from build123d import *

# Parameters (mm, degrees)
F0_R     = 3
F1_DEPTH = 6
F2_R     = 8.6602540378
F3_DEPTH = 6
F4_R     = 5.99999
F5_R     = 0.75
F6_DEPTH = 3
F7_R     = 3
F8_DEPTH = 101
F10_R    = 2.5
F11_R    = 3


# Not quite as in the source:
# - a fillet or chamfer is up to 0.001 mm smaller than in the source, because OpenCascade refuses the exact size


with BuildPart() as f1:
    # F0 (on Top) → F1 (new body)
    with BuildSketch(Plane.XY):
        Polygon((5, 8.6602540378), (-5, 8.6602540378), (-10, 0), (-5, -8.6602540378), (5, -8.6602540378), (10, 0), align=None)
        Circle(F0_R, mode=Mode.SUBTRACT)
        Circle(F0_R)
    extrude(amount=F1_DEPTH)

    # F2 (on face) → F3 (join)
    with BuildSketch(Plane.XY.offset(6)):
        Circle(F2_R)
    extrude(amount=F3_DEPTH)

    # F4 (radius 6 in the source; OpenCascade refuses exactly that, so slightly less here)
    f4_edges = [f1.edges().sort_by_distance(p)[0] for p in [
        (-8.660254, 0, 12),
    ]]
    fillet(f4_edges, radius=F4_R)

    # F5 (on face) → F6 (cut)
    with BuildSketch(Plane.XY.offset(12)):
        Circle(F5_R)
    extrude(amount=-F6_DEPTH, mode=Mode.SUBTRACT)

    # F7 (on face) → F8 (join)
    with BuildSketch(Plane(origin=(0, 0, 0), x_dir=(1, 0, 0), z_dir=(0, 0, -1))):
        Circle(F7_R)
    extrude(amount=F8_DEPTH)

    # F10 (on offset) → F12 section 0
    with BuildSketch(Plane(origin=(0, 0, -109), x_dir=(1, 0, 0), z_dir=(0, 0, -1))):
        Circle(F10_R)
    # F11 (on face) → F12 section 1
    with BuildSketch(Plane(origin=(0, 0, -101), x_dir=(1, 0, 0), z_dir=(0, 0, -1))):
        Circle(F11_R)
    loft()


solid = f1.part
Here's how the part is built. I have some questions about the finished solid (model axes, mm). A direction names the side the tool comes from. Coordinates: 2 decimals unless noted, no trailing zeros. Write each loop counter-clockwise with the first axis right and the second up, starting at its lowest first coordinate (ties: lowest second). Pieces come first, ordered by that corner, then holes.
Item 1: On a 3-axis mill with a long thin cutter (end or side, diameter ignored), from which of +Z, -Z, +X, -X, +Y, -Y can I reach the whole of each face in a straight line? I mean faces 1 (the flat face through (-4, 8, 6)), 2 (the flat face through (0, 4, 0)), 3 (the flat face through (5, 8, 6)). Say none if no direction works.
Item 2: I want a section at A-A on z = -97. Write out the boundary of the cut face in (x, y), and give its area (3 significant figures).
Item 3: If I drill on line 1 (Y direction, x = 0, z = 11.2); line 2 (Y direction, x = 0, z = 9.7); line 3 (Z direction, x = 7.25, y = -3.75), over which ranges is the centre line in solid material (lowest first)?
Item 4: Will these pins go through, and if not, where does the flat tip stop? pin 1 (10 mm diameter, centred on x = -3, z = -76, fed in from +Y); pin 2 (1.3 mm diameter, centred on x = 3.5, y = -6.5, fed in from +Z); pin 3 (3.5 mm diameter, centred on x = -4, y = -7, fed in from +Z); pin 4 (4 mm diameter, centred on y = 6.5, z = -14, fed in from -X).
Findings below:
1. face 1: +Z, -X, +Y
1. face 2: -Z
1. face 3: +Z, +X, +Y
2. outline: circle Ø6 at (0, 0)
2. area: 28.3 mm2
3. line 1: y = -5.65 to -0.75, 0.75 to 5.65
3. line 2: y = -7.38 to -0.75, 0.75 to 7.38
3. line 3: z = 0 to 8.39
4. pin 1: stops at y = 3
4. pin 2: stops at z = 10.41
4. pin 3: stops at z = 10.76
4. pin 4: passes through
